```python
from build123d import *

# Parameters (mm, degrees)
SKETCH1_W           = 150
SKETCH1_H           = 70
BOSS_EXTRUDE1_DEPTH = 4
SKETCH7_R           = 2
CUT_EXTRUDE2_DEPTH  = 30
BOSS_EXTRUDE7_START = -30
SKETCH4_R           = 12
SKETCH4_R_2         = 6
BOSS_EXTRUDE7_DEPTH = 30
LPATTERN2_COUNT     = 2
LPATTERN2_PITCH     = 60
CHAMFER3_SIZE       = 4
SKETCH8_W           = 30
SKETCH8_H           = 6.046246811
CUT_EXTRUDE3_DEPTH  = 10
SKETCH9_W           = 30
SKETCH9_H           = 6.046246811
CUT_EXTRUDE4_DEPTH  = 10
SKETCH10_W          = 30
SKETCH10_H          = 5.803707669
CUT_EXTRUDE5_DEPTH  = 10


with BuildPart() as part:
    # Sketch1 → Boss-Extrude1 (new body, symmetric)
    with BuildSketch(Plane.XY):
        Rectangle(SKETCH1_W, SKETCH1_H)
    extrude(amount=BOSS_EXTRUDE1_DEPTH, both=True)

    # Sketch7 → Cut-Extrude2 (cut)
    with BuildSketch(Plane.XY.offset(4)):
        with Locations((-56.630501899, 15.015863732)):
            Circle(SKETCH7_R)
        with Locations((0, -21.058085924)):
            Circle(SKETCH7_R)
        with Locations((61.669656729, 15.015863732)):
            Circle(SKETCH7_R)
    extrude(amount=-CUT_EXTRUDE2_DEPTH, mode=Mode.SUBTRACT)

    # Sketch4 → Boss-Extrude7 (add)
    with BuildSketch(Plane(origin=(75, 0, 0), x_dir=(0, 0, -1), z_dir=(1, 0, 0)).offset(BOSS_EXTRUDE7_START)):
        with Locations((6.400440408, 40.953753189)):
            Circle(SKETCH4_R)
        with Locations((6.400440408, 40.953753189)):
            Circle(SKETCH4_R_2, mode=Mode.SUBTRACT)
    boss_extrude7 = extrude(amount=-BOSS_EXTRUDE7_DEPTH)

    # LPattern2: Boss-Extrude7 ×2
    with Locations(*[(-i * LPATTERN2_PITCH, 0, 0) for i in range(1, LPATTERN2_COUNT)]):
        add(boss_extrude7)

    # Chamfer3
    chamfer3_edges = [part.edges().sort_by_distance(p)[0] for p in [
        (-58.630501899, 15.015863732, -4),
        (-2, -21.058085924, -4),
        (59.669656729, 15.015863732, -4),
    ]]
    chamfer(chamfer3_edges, length=CHAMFER3_SIZE)

    # Sketch8 → Cut-Extrude3 (cut)
    with BuildSketch(Plane.XY.offset(4)):
        with Locations((60, 31.976876594)):
            Rectangle(SKETCH8_W, SKETCH8_H)
    extrude(amount=-CUT_EXTRUDE3_DEPTH, mode=Mode.SUBTRACT)

    # Sketch9 → Cut-Extrude4 (cut)
    with BuildSketch(Plane(origin=(0, 0, -4), x_dir=(-1, 0, 0), z_dir=(0, 0, -1))):
        with Locations((60, 31.976876594)):
            Rectangle(SKETCH9_W, SKETCH9_H)
    extrude(amount=-CUT_EXTRUDE4_DEPTH, mode=Mode.SUBTRACT)

    # Sketch10 → Cut-Extrude5 (cut)
    with BuildSketch(Plane(origin=(0, 0, -4), x_dir=(-1, 0, 0), z_dir=(0, 0, -1))):
        with Locations((0, 32.098146165)):
            Rectangle(SKETCH10_W, SKETCH10_H)
    extrude(amount=-CUT_EXTRUDE5_DEPTH, mode=Mode.SUBTRACT)


solid = part.part
```
The listing builds one solid part. Answer for the finished solid, in the listing's coordinates (mm). A direction names the side the tool comes from. Give positions to 0.01 mm unless a question says otherwise; leave off trailing zeros. Order: outer loops, then holes, each group sorted by start corner. A loop starts at its lowest first (then second) coordinate and runs counter-clockwise, first axis right, second up.
Item 1: Which of the six approach directions +Z, -Z, +X, -X, +Y, -Y give full straight-line access (tool end or side, diameter ignored) to faces 5 (the face through (0, 29.196, 0)), 6 (the face through (-1, 0, 4)), 7 (the face through (-45, 35, -4))?
From the geometry:
face 5: +Z, -Z, +Y
face 6: +Z, +X, -X, -Y
face 7: +Z, -Z, -X, +Y
Item 2: The part is cut by section C-C, the plane z = -14.25. Give the vertices of the cut face in (x, y).
From the geometry:
outline: (-45, 31.88) - (-15, 31.88) - (-15, 50.03) - (-45, 50.03) - close; (15, 31.88) - (45, 31.88) - (45, 50.03) - (15, 50.03) - close
Item 3: Find the intervals of material crossed by probe 1 along Y at (x, z) = (0, 3); probe 2 along Z at (x, y) = (16.5, 41); probe 3 along X at (y, z) = (47, 1.75), in increasing order.
From the geometry:
probe 1: y = -35 to -23.06, -19.06 to 29.2
probe 2: z = -18.4 to -12.4, -0.4 to 5.6
probe 3: x = -45 to -15, 15 to 45
Item 4: For a pull along Y with two mould halves and no side action, classify faces 1 (the face through (-29.79, 35.096, -5.1)), 2 (the face through (45, 35, -4)), 3 (the face through (60, 28.954, 0)), 4 (the face through (-58.88, 15.11, -0.25)) as pulls with the +Y half, pulls with the -Y half, needs draft (parallel to the pull), parting line crosses it, or undercut.
From the geometry:
face 1: undercut
face 2: needs draft
face 3: pulls with the +Y half
face 4: undercut
Item 5: The part is cut by section D-D, the plane x = 26. Give the vertices of the cut face in (y, z), and give its area (3 significant figures).
From the geometry:
outline: (-35, -4) - (29.2, -4) arc R12 ccw (long way) to (34.97, 4) - (-35, 4) - close; hole circle Ø12 at (40.95, -6.4)
area: 869 mm2
Item 6: The part is cut by section B-B, the plane y = 37. Give the vertices of the cut face in (x, z), and give its area (3 significant figures).
From the geometry:
outline: (-45, -17.73) - (-15, -17.73) - (-15, -10.91) - (-45, -10.91) - close; (-45, -1.89) - (-15, -1.89) - (-15, 4.93) - (-45, 4.93) - close; (15, -17.73) - (45, -17.73) - (45, -10.91) - (15, -10.91) - close; (15, -1.89) - (45, -1.89) - (45, 4.93) - (15, 4.93) - close
area: 818 mm2
Item 7: The part is cut by section A-A, the plane x = 0. Give the vertices of the cut face in (y, z), and give its area (3 significant figures).
From the geometry:
outline: (-35, -4) - (-27.06, -4) - (-23.06, 0) - (-23.06, 4) - (-35, 4) - close; (-19.06, 0) - (-15.06, -4) - (29.2, -4) - (29.2, 4) - (-19.06, 4) - close
area: 466 mm2
Item 8: Given pin 1 Ø10 at (y, z) = (38, -6) entering from -X; pin 2 Ø4 at (x, z) = (-0.5, 0) entering from +Y; pin 3 Ø14 at (y, z) = (40.95, -6.4) entering from +X, each flat-ended and moving along its own axis, determine where each tip first touches the part or whether it passes through.
From the geometry:
pin 1: stops at x = -45
pin 2: stops at y = 29.2
pin 3: stops at x = 45
